CAD build for the part. Positions are in the model's coordinates, mm. Give positions to 0.01 mm unless a question says otherwise; leave off trailing zeros. Order: outer loops, then holes, each group sorted by start corner. A loop starts at its lowest first (then second) coordinate and runs counter-clockwise, first axis right, second up. Notation, with made-up numbers: (84.5, 10.5) -> (134.5, 10.5) arc R22 cw to (134.5, 23.5) -> close; hole circle Ø7 at (71.5, -3). An arc over 180 degrees is marked (long way). Answer as CSV lines item,"result".
```python
from build123d import *

# Parameters (mm, degrees)
SKETCH1_R           = 84.709
SKETCH1_R_2         = 78.359
BOSS_EXTRUDE1_DEPTH = 19.05
SKETCH2_R           = 3.478244762
CUT_EXTRUDE1_DEPTH  = 122.301821347
CIRPATTERN1_COUNT   = 6


with BuildPart() as part:
    # Sketch1 → Boss-Extrude1 (new body)
    with BuildSketch(Plane.XY):
        with Locations(Location((0, 0, 0), (0, 0, 180))):
            Circle(SKETCH1_R)
        with Locations(Location((0, 0, 0), (0, 0, 180))):
            Circle(SKETCH1_R_2, mode=Mode.SUBTRACT)
    extrude(amount=BOSS_EXTRUDE1_DEPTH)

    # Sketch2 → Cut-Extrude1 (cut, through all)
    with BuildSketch(Plane(origin=(0, 0, 0), x_dir=(1, 0, 0), z_dir=(0, 1, 0))):
        with Locations(Location((0, -9.525, 0), (0, 0, 270))):
            Circle(SKETCH2_R)
    cut_extrude1 = extrude(amount=-CUT_EXTRUDE1_DEPTH, mode=Mode.SUBTRACT)

    # CirPattern1: Cut-Extrude1 ×6 about axis
    cirpattern1_axis = Axis((0, 0, 2.080715754), (0, 0, 1))
    for i in range(1, CIRPATTERN1_COUNT):
        add(cut_extrude1.rotate(cirpattern1_axis, i * 360 / CIRPATTERN1_COUNT), mode=Mode.SUBTRACT)


solid = part.part
```
1) Band-saw the part on B-B, the plane y = 0. Write the cut outline in (x, z), then the cut area to 3 significant figures.
Data:
outline,"(-84.71, 0) -> (-78.36, 0) -> (-78.36, 19.05) -> (-84.71, 19.05) -> close; (78.36, 0) -> (84.71, 0) -> (84.71, 19.05) -> (78.36, 19.05) -> close"
area,"242 mm2"
2) Band-saw the part on D-D, the plane z = 17. Write the cut outline in (x, y).
Data:
outline,"circle Ø169.42 at (0, 0); hole circle Ø156.72 at (0, 0)"
3) Pin check, flat tips, straight feed: P1, Ø9, axis at x = 0, z = 9.525, coming from the +Y side; P2, Ø6, axis at y = -33.5, z = 13.5, coming from the +X side; P3, Ø4, axis at x = -24.5, z = 6, coming from the +Y side; P4, Ø2, axis at x = -61.5, z = 13.5, coming from the -Y side. Stop position of each tip, or through.
Data:
P1,"stops at y = 84.71"
P2,"stops at x = 79.03"
P3,"stops at y = 81.67"
P4,"stops at y = -59.29"
4) Band-saw the part on C-C, the plane x = 60. Write the cut outline in (y, z), then the cut area to 3 significant figures.
Data:
outline,"(-59.8, 0) -> (-50.4, 0) -> (-50.4, 19.05) -> (-59.8, 19.05) -> close; (50.4, 0) -> (59.8, 0) -> (59.8, 19.05) -> (50.4, 19.05) -> close"
area,"358 mm2"
5) Pull direction Y, two halves, no side cores. Call faces 1 (the cylindrical face through (-0.15, 81.45, 6.05)), 2 (the cylindrical face through (-80.8, -25.44, 9.39)), 3 (the cylindrical face through (68.84, -43.665, 8.771)): pulls with the +Y half, pulls with the -Y half, needs draft (parallel to the pull), parting line crosses it, or undercut.
Data:
face 1,"needs draft"
face 2,"parting line crosses it"
face 3,"undercut"
6) Wall check: line 1 along Z through (x, y) = (0, -82.75); line 2 along Y through (x, z) = (-1, 1); line 3 along Y through (x, z) = (-71, 10). Give the ranges that are in metal, low to high. Write a range as [from, to].
Data:
line 1,"z = [0, 6.05], [13, 19.05]"
line 2,"y = [-84.7, -78.35], [78.35, 84.7]"
line 3,"y = [-46.2, -44.97], [-37.01, -33.15], [33.15, 37.01], [44.97, 46.2]"
7) Band-saw the part on A-A, the plane x = 0. Write the cut outline in (y, z), then the cut area to 3 significant figures.
Data:
outline,"(-84.71, 0) -> (-78.36, 0) -> (-78.36, 6.05) -> (-84.71, 6.05) -> close; (-84.71, 13) -> (-78.36, 13) -> (-78.36, 19.05) -> (-84.71, 19.05) -> close; (78.36, 0) -> (84.71, 0) -> (84.71, 6.05) -> (78.36, 6.05) -> close; (78.36, 13) -> (84.71, 13) -> (84.71, 19.05) -> (78.36, 19.05) -> close"
area,"154 mm2"
